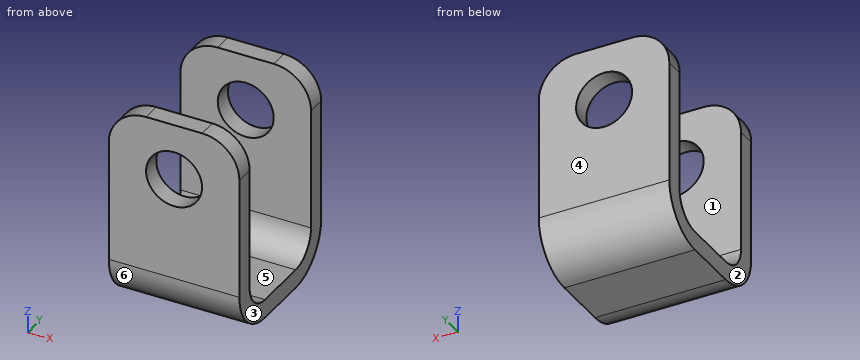
```python
from build123d import *

# Parameters (mm, degrees)
SKETCH12_W                     = 22.225
SKETCH12_H                     = 25.4
BASE_FLANGE2_DEPTH             = 3.175
EDGE_FLANGE2_STRIP_W           = 22.225
EDGE_FLANGE2_STRIP_H           = 3.175
EDGE_FLANGE2_STRIP_CUT_DEPTH   = 22.225
EDGE_FLANGE2_STRIP_2_W         = 22.225
EDGE_FLANGE2_STRIP_2_H         = 3.175
EDGE_FLANGE2_STRIP_CUT_2_DEPTH = 22.225
EDGE_FLANGE2_DEPTH             = 22.225
EDGE_FLANGE2_BEND_DEPTH        = 22.225
CUT_EXTRUDE1_DEPTH             = 53.098064084
CUT_EXTRUDE1_DEPTH_BACK        = 53.098064084
SKETCH23_R                     = 4.7625
BREAK_CORNER1_START            = -12.7
BREAK_CORNER1_DEPTH            = 25.4


# Read off the part's stored shape, not the designer's step: Break-Corner1
# Sheet-metal steps are written as plain solids
with BuildPart() as part:
    # Sketch12 → Base-Flange2 (new body)
    with BuildSketch(Plane.XY):
        with Locations((25.4, 0)):
            Rectangle(SKETCH12_W, SKETCH12_H)
    extrude(amount=BASE_FLANGE2_DEPTH)

    # Edge-Flange2 strip (across the edge) → Edge-Flange2 strip cut (cut)
    with BuildSketch(Plane(origin=(36.5125, 12.7, 3.175), x_dir=(0, -1, 0), z_dir=(-1, 0, 0))):
        with Locations((-3.175, -1.5875)):
            Rectangle(EDGE_FLANGE2_STRIP_W, EDGE_FLANGE2_STRIP_H)
    extrude(amount=EDGE_FLANGE2_STRIP_CUT_DEPTH, mode=Mode.SUBTRACT)

    # Edge-Flange2 strip 2 (across the edge) → Edge-Flange2 strip cut 2 (cut)
    with BuildSketch(Plane(origin=(14.2875, -12.7, 3.175), x_dir=(0, 1, 0), z_dir=(1, 0, 0))):
        with Locations((-3.175, -1.5875)):
            Rectangle(EDGE_FLANGE2_STRIP_2_W, EDGE_FLANGE2_STRIP_2_H)
    extrude(amount=EDGE_FLANGE2_STRIP_CUT_2_DEPTH, mode=Mode.SUBTRACT)

    # Edge-Flange2 section (across the edge) → Edge-Flange2 (add)
    with BuildSketch(Plane(origin=(36.5125, 12.7, 3.175), x_dir=(0, -1, 0), z_dir=(-1, 0, 0))):
        with BuildLine():
            Line((0, 4.7625), (0, 31.75))
            Line((0, 31.75), (3.175, 31.75))
            Line((3.175, 31.75), (3.175, 4.7625))
            ThreePointArc((3.175, 4.7625), (4.569903955, 1.394903955), (7.9375, 0))
            Line((7.9375, 0), (7.9375, -3.175))
            ThreePointArc((7.9375, -3.175), (2.324839924, -0.850160076), (0, 4.7625))
        make_face()
    extrude(amount=EDGE_FLANGE2_DEPTH)

    # Edge-Flange2 section 2 (across the edge) → Edge-Flange2 bend (add)
    with BuildSketch(Plane(origin=(14.2875, -12.7, 3.175), x_dir=(0, 1, 0), z_dir=(1, 0, 0))):
        with BuildLine():
            Line((0, 4.7625), (0, 31.75))
            Line((0, 31.75), (3.175, 31.75))
            Line((3.175, 31.75), (3.175, 4.7625))
            ThreePointArc((3.175, 4.7625), (4.569903955, 1.394903955), (7.9375, 0))
            Line((7.9375, 0), (7.9375, -3.175))
            ThreePointArc((7.9375, -3.175), (2.324839924, -0.850160076), (0, 4.7625))
        make_face()
    extrude(amount=EDGE_FLANGE2_BEND_DEPTH)

    # Sketch23 → Cut-Extrude1 (cut, two sides: drawn at the far end of the back side and taken through both)
    with BuildSketch(Plane(origin=(0, 0, 0), x_dir=(1, 0, 0), z_dir=(0, 1, 0)).offset(-CUT_EXTRUDE1_DEPTH_BACK)):
        with Locations(Location((25.4, -25.4, 0), (0, 0, 270))):
            Circle(SKETCH23_R)
    extrude(amount=CUT_EXTRUDE1_DEPTH + CUT_EXTRUDE1_DEPTH_BACK, mode=Mode.SUBTRACT)

    # Break-Corner1 outline → Break-Corner1 (cut)
    with BuildSketch(Plane(origin=(0, 0, 0), x_dir=(1, 0, 0), z_dir=(0, 1, 0)).offset(BREAK_CORNER1_START)):
        with BuildLine():
            Line((36.5125, -34.925), (36.5125, -28.575))
            ThreePointArc((36.5125, -28.575), (34.652628061, -33.065128061), (30.1625, -34.925))
            Line((30.1625, -34.925), (36.5125, -34.925))
        make_face()
        with BuildLine():
            Line((14.2875, -34.925), (20.6375, -34.925))
            ThreePointArc((20.6375, -34.925), (16.147371939, -33.065128061), (14.2875, -28.575))
            Line((14.2875, -28.575), (14.2875, -34.925))
        make_face()
    extrude(amount=BREAK_CORNER1_DEPTH, mode=Mode.SUBTRACT)


solid = part.part
```
Geometry check sheet. Reference: the model listing, model coordinates, mm. Face numbers are marked on the shaded views. A direction names the side the tool comes from. Give positions to 0.01 mm unless a question says otherwise; leave off trailing zeros. Order: outer loops, then holes, each group sorted by start corner. A loop starts at its lowest first (then second) coordinate and runs counter-clockwise, first axis right, second up.
1. Release check for a two-part mould opening along Y. For the marked faces 3, 4, 5 and 6 record: pulls with the +Y half, pulls with the -Y half, needs draft (parallel to the pull), parting line crosses it, or undercut.
2. Thickness scan on L1, parallel to X at y = -11.15, z = 25.4; L2, parallel to Y at x = 29, z = 19 (3 decimals); L3, parallel to Z at x = 28, y = 4.75 (3 decimals). Record the ranges inside material, lowest first.
3. Gauge pin test, flat ends, axial feed: pin 1 Ø4 at (x, y) = (21.5, -6) entering from +Z; pin 2 Ø5 at (x, y) = (30.5, 2) entering from +Z (3 decimals); pin 3 Ø1.5 at (x, z) = (20, 4) entering from +Y. Record the tip position at first contact, or that the pin passes through.
4. Section check A-A, the plane x = 25.4. Enter the section's corners in (y, z) (1 decimal), and give its area (3 significant figures).
5. Section check B-B, the plane z = 19.5. Enter the section's corners in (x, y) (1 decimal).
6. Section check C-C, the plane z = 25.4. Enter the section's corners in (x, y) (1 decimal), and give its area (3 significant figures).
7. Access from +Z, -Z, +X, -X, +Y, -Y to the whole of each face (thin tool, end or side, straight path). Record for the marked faces 1 and 2.
Values follow:
1. face 3: needs draft
1. face 4: pulls with the +Y half
1. face 5: undercut
1. face 6: pulls with the -Y half
2. L1: x = 14.29 to 20.64, 30.16 to 36.51
2. L2: y = -12.7 to -9.525, 9.525 to 12.7
2. L3: z = 0 to 3.175
3. pin 1: stops at z = 4.44
3. pin 2: stops at z = 3.175
3. pin 3: stops at y = 12.03
4. outline: (-12.7, 7.9) arc R7.9 ccw to (-4.8, 0) - (4.8, 0) arc R7.9 ccw to (12.7, 7.9) - (12.7, 20.6) - (9.5, 20.6) - (9.5, 7.9) arc R4.8 cw to (4.8, 3.2) - (-4.8, 3.2) arc R4.8 cw to (-9.5, 7.9) - (-9.5, 20.6) - (-12.7, 20.6) - close; (-12.7, 30.2) - (-9.5, 30.2) - (-9.5, 34.9) - (-12.7, 34.9) - close; (9.5, 30.2) - (12.7, 30.2) - (12.7, 34.9) - (9.5, 34.9) - close
4. area: 204 mm2
5. outline: (14.3, -12.7) - (36.5, -12.7) - (36.5, -9.5) - (14.3, -9.5) - close; (14.3, 9.5) - (36.5, 9.5) - (36.5, 12.7) - (14.3, 12.7) - close
6. outline: (14.3, -12.7) - (20.6, -12.7) - (20.6, -9.5) - (14.3, -9.5) - close; (14.3, 9.5) - (20.6, 9.5) - (20.6, 12.7) - (14.3, 12.7) - close; (30.2, -12.7) - (36.5, -12.7) - (36.5, -9.5) - (30.2, -9.5) - close; (30.2, 9.5) - (36.5, 9.5) - (36.5, 12.7) - (30.2, 12.7) - close
6. area: 80.6 mm2
7. face 1: +Z, +X, -X
7. face 2: +Z, -Z, -X, +Y, -Y
